Answer from the drawing. Dimensions are ordinates in mm from the lowest x, y and z of the part. Give positions to 0.01 mm unless a question says otherwise; leave off trailing zeros. Write each loop counter-clockwise with the first axis right and the second up, starting at its lowest first coordinate (ties: lowest second). Pieces come first, ordered by that corner, then holes. Notation, with made-up numbers: (56, 10) - (61, 10) arc R15 ccw to (61, 32) - close; hole circle Ø11 at (1.25, -22.75). An arc over 180 degrees is marked (long way). Write item = value, one per line.
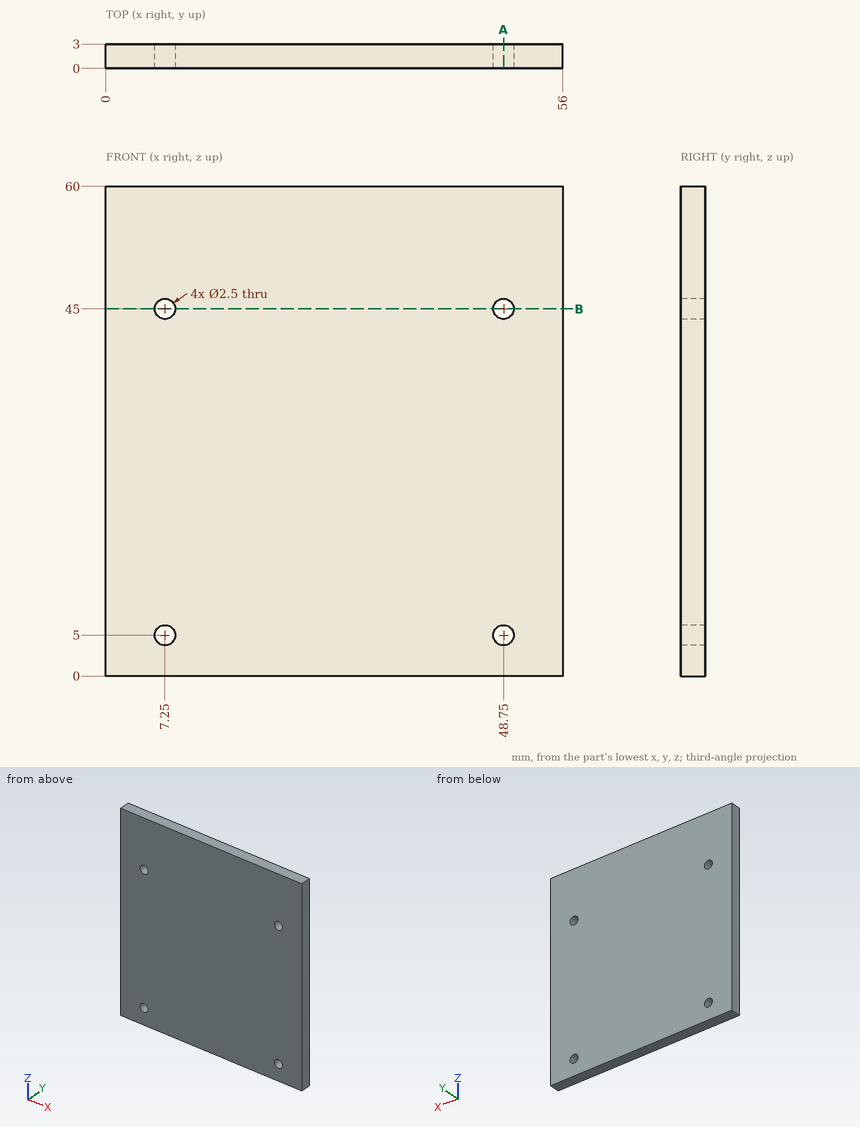
1. Straight lines are drawn through the part: line 1 (Z direction, x = 7.25, y = 1); line 2 (Z direction, x = 8, y = 2.7). For each, find the intervals that lie inside material, in ascending order.
Solution:
line_1 = 0 to 3.75, 6.25 to 43.75, 46.25 to 60
line_2 = 0 to 4, 6 to 44, 46 to 60
2. Find section A-A, the plane x = 48.75. Give the vertices of the cut face in (y, z), then the cut area to 3 significant figures.
Solution:
outline = (0, 0) - (3, 0) - (3, 3.75) - (0, 3.75) - close; (0, 6.25) - (3, 6.25) - (3, 43.75) - (0, 43.75) - close; (0, 46.25) - (3, 46.25) - (3, 60) - (0, 60) - close
area = 165 mm^2
3. Find section B-B, the plane z = 45. Give the vertices of the cut face in (x, y), then the cut area to 3 significant figures.
Solution:
outline = (0, 0) - (6, 0) - (6, 3) - (0, 3) - close; (8.5, 0) - (47.5, 0) - (47.5, 3) - (8.5, 3) - close; (50, 0) - (56, 0) - (56, 3) - (50, 3) - close
area = 153 mm^2
4. Given pin 1 (1 mm diameter, centred on x = 30.5, y = 2, fed in from -Z), flat-ended and moving along its own axis, determine where the tip first touches the part or whether it passes through.
Solution:
pin_1 = 0
